The model under review builds one solid part; all positions refer to its coordinate system, in mm. A direction names the side the tool comes from. Give positions to 0.01 mm unless a question says otherwise; leave off trailing zeros. Loops run counter-clockwise (first coordinate to the right, second up) from the corner with the lowest first, then second, coordinate; pieces in that order, holes last. Notation, with made-up numbers: (-27.5, 19.5) - (31.5, 19.5) arc R23 ccw to (31.5, 43.5) - close; hole circle Ø1 at (52, 32). An arc over 180 degrees is marked (long way). Return JSON: item names as keys, results as strings. Group by question number.
from build123d import *

# Parameters (mm, degrees)
F1_DEPTH = 82
F2_R     = 14
F3_R     = 5.5
F4_DEPTH = 16.001
F5_R     = 3


with BuildPart() as f1:
    # F0 (on Front) → F1 (new body)
    with BuildSketch(Plane.XZ):
        Polygon((0, 12), (0, 0), (38, 0), (38, -4), (103.254273, -4), (103.254273, 0), (141.254273, 0), (141.254273, 12), (97.254273, 12), (97.254273, 8), (44, 8), (44, 12), align=None)
    extrude(amount=F1_DEPTH)

    # F2
    f2_edges = [f1.edges().sort_by_distance(p)[0] for p in [
        (141.254273, -82, 6),
        (141.254273, 0, 6),
        (0, -82, 6),
        (0, 0, 6),
    ]]
    fillet(f2_edges, radius=F2_R)

    # F3 (on face) → F4 (cut, through all)
    with BuildSketch(Plane.XY.offset(12)):
        with Locations((128.337874, -68)):
            Circle(F3_R)
        with Locations((128.337874, -14)):
            Circle(F3_R)
        with Locations((14, -68)):
            Circle(F3_R)
        with Locations((14, -14)):
            Circle(F3_R)
    extrude(amount=-F4_DEPTH, mode=Mode.SUBTRACT)

    # F5
    f5_edges = [f1.edges().sort_by_distance(p)[0] for p in [
        (44, -41, 8),
        (97.254273, -41, 8),
    ]]
    fillet(f5_edges, radius=F5_R)


solid = f1.part
Item 1: Tool access review of faces 4 (the face through (19.08, -16.11, 6.08)), 5 (the face through (44.86, -41.57, 8.9)), 6 (the face through (19, -40, 0)): name each direction out of +Z, -Z, +X, -X, +Y, -Y from which nothing blocks a thin tool from reaching the whole face with its end or side.
Item 2: Mouldability with a two-part tool opening along X and no side actions: class faces 1 (the face through (70, -40, -4)), 2 (the face through (103.254, -40, -2)), 3 (the face through (133.418, -16.107, 6.084)) as +X half, -X half, draft (parallel to the pull), parting line (faces both ways), or undercut.
Item 3: Take a section at C-C (y = -23.5). State the section outline as (x, z) points, then the cut area to 3 significant figures.
Item 4: Take a section at A-A (z = 2). State the section outline as (x, y) points.
Item 5: Take a section at B-B (y = -12). State the section outline as (x, z) points, then the cut area to 3 significant figures.
Item 6: For L1, parallel to Y at x = 14, z = 7.5; L2, parallel to Y at x = 15.5, z = 9; L3, parallel to Z at x = 85, y = -37, list the stretches that pass through material, from the lowest coordinate up. Write a range as from..to.
Item 7: For P1, Ø17.5, axis at x = 128.34, y = -68, coming from the +Z side; P2, Ø10, axis at x = 128.34, y = -14, coming from the +Z side; P3, Ø2, axis at y = -34, z = -2.5, coming from the +X side; P4, Ø1, axis at x = 35.5, y = -23, coming from the -Z side, all flat-tipped, find the tip position at first contact; note any pin that passes through.
Item 8: Take a section at D-D (x = 35.5). State the section outline as (y, z) points, then the cut area to 3 significant figures.
Check sheet entries:
{
 "1": {"face 4": "+Z, -Z", "face 5": "+Z, +Y, -Y", "face 6": "-Z, -X, +Y, -Y"},
 "2": {"face 1": "draft", "face 2": "+X half", "face 3": "undercut"},
 "3": {"outline": "(0, 0) - (38, 0) - (38, -4) - (103.25, -4) - (103.25, 0) - (141.25, 0) - (141.25, 12) - (97.25, 12) - (97.25, 11) arc R3 cw to (94.25, 8) - (47, 8) arc R3 cw to (44, 11) - (44, 12) - (0, 12) - close", "area": "1,750 mm^2"},
 "4": {"outline": "(0, -68) arc R14 ccw to (14, -82) - (127.25, -82) arc R14 ccw to (141.25, -68) - (141.25, -14) arc R14 ccw to (127.25, 0) - (14, 0) arc R14 ccw to (0, -14) - close; hole circle Ø11 at (14, -68); hole circle Ø11 at (14, -14); hole circle Ø11 at (128.34, -68); hole circle Ø11 at (128.34, -14)"},
 "5": {"outline": "(0.14, 0) - (8.88, 0) - (8.88, 12) - (0.14, 12) - close; (19.12, 0) - (38, 0) - (38, -4) - (103.25, -4) - (103.25, 0) - (123.21, 0) - (123.21, 12) - (97.25, 12) - (97.25, 11) arc R3 cw to (94.25, 8) - (47, 8) arc R3 cw to (44, 11) - (44, 12) - (19.12, 12) - close; (133.46, 0) - (141.11, 0) - (141.11, 12) - (133.46, 12) - close", "area": "1,500 mm^2"},
 "6": {"L1": "y = -82..-73.5, -62.5..-19.5, -8.5..0", "L2": "y = -82..-73.29, -62.71..-19.29, -8.71..0", "L3": "z = -4..8"},
 "7": {"P1": "stops at z = 12", "P2": "passes through", "P3": "stops at x = 103.25", "P4": "stops at z = 0"},
 "8": {"outline": "(-82, 0) - (0, 0) - (0, 12) - (-82, 12) - close", "area": "984 mm^2"}
}
